```python
from build123d import *

# Parameters (mm, degrees)
F1_DEPTH = 63.5
F0_W     = 25.4
F0_H     = 19.05
F2_DEPTH = 25.4
F3_DEPTH = 7.9375
F5_R     = 6.35
F6_R     = 11.7795473759
F7_DEPTH = 28.575


with BuildPart() as f1:
    # F0 (on Front) → F1 (new body, symmetric)
    with BuildSketch(Plane.XZ):
        Polygon((-41.275, 9.525), (-41.275, -9.525), (41.275, -9.525), (41.275, 9.525), (22.225, 9.525), align=None)
    extrude(amount=F1_DEPTH, both=True)

    # F0 (on Front) → F2 (join, symmetric)
    with BuildSketch(Plane.XZ):
        with BuildLine():
            Line((22.225, 9.525), (41.275, 9.525))
            Line((41.275, 9.525), (41.275, 27.0002))
            ThreePointArc((41.275, 27.0002), (45.9246798487, 38.2255201513), (57.15, 42.8752))
            Line((57.15, 42.8752), (60.325, 42.8752))
            Line((60.325, 42.8752), (60.325, 61.9252))
            Line((60.325, 61.9252), (57.15, 61.9252))
            ThreePointArc((57.15, 61.9252), (32.4542956671, 51.6959043329), (22.225, 27.0002))
            Line((22.225, 27.0002), (22.225, 9.525))
        make_face()
        with Locations((73.025, 52.4002)):
            Rectangle(F0_W, F0_H)
    extrude(amount=F2_DEPTH, both=True)

    # F0 (on Front) → F3 (join, symmetric)
    with BuildSketch(Plane.XZ):
        with BuildLine():
            add(Edge.make_bspline(
                [(-41.275, 9.525), (-41.275, 29.0132258087), (19.6397230029, 61.9252), (57.15, 61.9252)],
                knots=[0, 0, 0, 0, 111.5045361635, 111.5045361635, 111.5045361635, 111.5045361635], degree=3))
            Line((-41.275, 9.525), (22.225, 9.525))
            Line((22.225, 9.525), (22.225, 27.0002))
            ThreePointArc((22.225, 27.0002), (32.4542956671, 51.6959043329), (57.15, 61.9252))
        make_face()
    extrude(amount=F3_DEPTH, both=True)

    # F0 (on Front) → F4 (revolve)
    with BuildSketch(Plane.XZ):
        Polygon((85.725, 66.675), (85.725, 61.9252), (85.725, 42.8752), (85.725, 38.1), (111.125, 38.1), (111.125, 66.675), align=None)
    revolve(axis=Axis((85.725, 0, 52.3875), (0, 0, 1)))

    # F5
    f5_edges = [f1.edges().sort_by_distance(p)[0] for p in [
        (41.275, -63.5, 0),
        (-41.275, -63.5, 0),
        (-41.275, 63.5, 0),
        (41.275, 63.5, 0),
    ]]
    fillet(f5_edges, radius=F5_R)

    # F6 (on face) → F7 (cut, through all)
    with BuildSketch(Plane.XY.offset(66.675)):
        with Locations((85.725, 0)):
            Circle(F6_R)
    extrude(amount=-F7_DEPTH, mode=Mode.SUBTRACT)


solid = f1.part
```
Model file for the job. Use its own axes, mm. A direction names the side the tool comes from. Round coordinates to 2 decimals unless told otherwise and drop trailing zeros. Write each loop counter-clockwise with the first axis right and the second up, starting at its lowest first coordinate (ties: lowest second). Pieces come first, ordered by that corner, then holes. Notation, with made-up numbers: (58.25, -30.5) - (95.25, -30.5) arc R29 cw to (95.25, -1.5) - close; hole circle Ø6 at (78.25, 27.5). An arc over 180 degrees is marked (long way). Use CSV: the item, a comma, the result in double quotes. Start each with the question number.
Item 1: Band-saw the part on D-D (y = 17). Write the cut outline in (x, z) (3 decimals).
Item 2: Band-saw the part on A-A (y = -14). Write the cut outline in (x, z) (3 decimals).
Item 3: Pin check, flat tips, straight feed: P1, Ø15.5, axis at x = 65, z = 34, coming from the -Y side; P2, Ø2, axis at x = 80.5, z = 43.5, coming from the -Y side; P3, Ø1.5, axis at y = -47, z = 6, coming from the +X side (3 decimals). Stop position of each tip, or through.
Item 4: Band-saw the part on B-B (x = 62.5). Write the cut outline in (y, z) (3 decimals), and give its area (3 significant figures).
Item 5: Drill centre lines: L1, parallel to Y at x = 51, z = 61.5; L2, parallel to Z at x = 3, y = 13.5 (3 decimals); L3, parallel to X at y = 9, z = 46. Where is each one in solid material? Low to high. Write a range as [from, to].
Item 6: Band-saw the part on C-C (y = -40). Write the cut outline in (x, z) (3 decimals), and give its area (3 significant figures).
Item 7: Two-plate mould, pull along X, no slides. Class faces 4 (the face through (96.96, 3.54, 52.59)), 5 (the face through (45.8, -0.4, 38.1)), 6 (the face through (41.275, -1, 4)), 7 (the face through (74.8, -5.3, 38.1)): released by +X, released by -X, zero draft, split by the parting line, or undercut.
Item 8: Tool access for faces 1 (the face through (22.225, -17, 18)), 2 (the face through (32.73, 16.55, 51.97)), 3 (the face through (60, -2, 61.925)): list every direction of +Z, -Z, +X, -X, +Y, -Y with a clear straight run to the whole face (end or side of a thin tool).
Checked values:
1,outline,"(-41.275, -9.525) - (41.275, -9.525) - (41.275, 27) arc R15.875 cw to (57.15, 42.875) - (66.853, 42.875) - (66.853, 38.1) - (104.597, 38.1) - (104.597, 66.675) - (66.853, 66.675) - (66.853, 61.925) - (57.15, 61.925) arc R34.925 ccw to (22.225, 27) - (22.225, 9.525) - (-41.275, 9.525) - close"
2,outline,"(-41.275, -9.525) - (41.275, -9.525) - (41.275, 27) arc R15.875 cw to (57.15, 42.875) - (64.532, 42.875) - (64.532, 38.1) - (106.918, 38.1) - (106.918, 66.675) - (64.532, 66.675) - (64.532, 61.925) - (57.15, 61.925) arc R34.925 ccw to (22.225, 27) - (22.225, 9.525) - (-41.275, 9.525) - close"
3,P1,"stops at y = -21.09"
3,P2,"stops at y = -25.4"
3,P3,"stops at x = 41.275"
4,outline,"(-25.4, 42.875) - (-10.284, 42.875) - (-10.284, 38.1) - (10.284, 38.1) - (10.284, 42.875) - (25.4, 42.875) - (25.4, 61.925) - (10.284, 61.925) - (10.284, 66.675) - (-10.284, 66.675) - (-10.284, 61.925) - (-25.4, 61.925) - close"
4,area,"1,160 mm²"
5,L1,"y = [-7.94, 7.94]"
5,L2,"z = [-9.525, 9.525]"
5,L3,"x = [27.85, 78.13], [93.32, 109.48]"
6,outline,"(-41.275, -9.525) - (41.275, -9.525) - (41.275, 9.525) - (-41.275, 9.525) - close"
6,area,"1,570 mm²"
7,face 4,"undercut"
7,face 5,"undercut"
7,face 6,"released by +X"
7,face 7,"zero draft"
8,face 1,"+Z, -X, -Y"
8,face 2,"+Z, -X, +Y"
8,face 3,"+Z, -X"
